CAD build for the part. Positions are in the model's coordinates, mm. Face numbers are marked on the shaded views. A direction names the side the tool comes from. Coordinates: 2 decimals unless noted, no trailing zeros. Order: outer loops, then holes, each group sorted by start corner. A loop starts at its lowest first (then second) coordinate and runs counter-clockwise, first axis right, second up. Notation, with made-up numbers: (43.25, -34.75) - (72.25, -34.75) arc R22 cw to (72.25, -3.75) - close; hole circle Ø7 at (-12.75, -10.5). An arc over 180 degrees is marked (long way). Return JSON: item names as keys, results as strings.
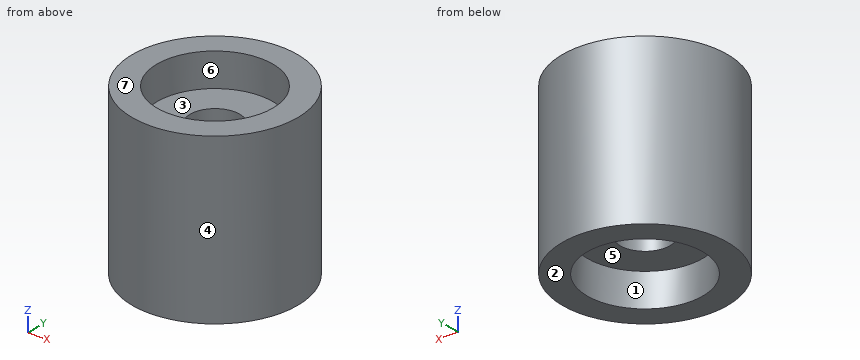
from build123d import *

# Parameters (mm, degrees)
SKETCH1_R           = 5
BOSS_EXTRUDE1_DEPTH = 10
SKETCH2_R           = 3.5
CUT_EXTRUDE1_DEPTH  = 2
SKETCH3_R           = 3.5
CUT_EXTRUDE2_DEPTH  = 2
SKETCH4_R           = 1.5
CUT_EXTRUDE3_DEPTH  = 12


with BuildPart() as part:
    # Sketch1 → Boss-Extrude1 (new body)
    with BuildSketch(Plane.XY):
        Circle(SKETCH1_R)
    extrude(amount=BOSS_EXTRUDE1_DEPTH)

    # Sketch2 → Cut-Extrude1 (cut)
    with BuildSketch(Plane.XY):
        Circle(SKETCH2_R)
    extrude(amount=CUT_EXTRUDE1_DEPTH, mode=Mode.SUBTRACT)

    # Sketch3 → Cut-Extrude2 (cut)
    with BuildSketch(Plane.XY.offset(10)):
        Circle(SKETCH3_R)
    extrude(amount=-CUT_EXTRUDE2_DEPTH, mode=Mode.SUBTRACT)

    # Sketch4 → Cut-Extrude3 (cut)
    with BuildSketch(Plane.XY.offset(10)):
        Circle(SKETCH4_R)
    extrude(amount=-CUT_EXTRUDE3_DEPTH, mode=Mode.SUBTRACT)


solid = part.part
Item 1: Band-saw the part on D-D, the plane y = -3.25. List the corners of the cut face in (x, z), then the cut area to 3 significant figures.
Findings below:
{"outline": "(-3.8, 0) - (-1.3, 0) - (-1.3, 2) - (1.3, 2) - (1.3, 0) - (3.8, 0) - (3.8, 10) - (1.3, 10) - (1.3, 8) - (-1.3, 8) - (-1.3, 10) - (-3.8, 10) - close", "area": "65.6 mm²"}
Item 2: Mould opens along Y. For the marked faces 4, 5, 6 and 7 say: released by +Y, released by -Y, zero draft, split by the parting line, or undercut.
Findings below:
{"face 4": "split by the parting line", "face 5": "undercut", "face 6": "undercut", "face 7": "zero draft"}
Item 3: Band-saw the part on A-A, the plane x = 0. List the corners of the cut face in (y, z).
Findings below:
{"outline": "(-5, 0) - (-3.5, 0) - (-3.5, 2) - (-1.5, 2) - (-1.5, 8) - (-3.5, 8) - (-3.5, 10) - (-5, 10) - close; (1.5, 2) - (3.5, 2) - (3.5, 0) - (5, 0) - (5, 10) - (3.5, 10) - (3.5, 8) - (1.5, 8) - close"}
Item 4: Band-saw the part on C-C, the plane z = 8.25. List the corners of the cut face in (x, y), then the cut area to 3 significant figures.
Findings below:
{"outline": "circle Ø10 at (0, 0); hole circle Ø7 at (0, 0)", "area": "40.1 mm²"}
Item 5: Drop flat-ended pins along their axis: P1, Ø2, axis at x = -1, y = -1.5, coming from the -Z side; P2, Ø2.5, axis at x = 0, y = 0, coming from the +Z side; P3, Ø1, axis at x = -3.5, z = 3.5, coming from the +Y side; P4, Ø1, axis at x = 2, z = 4.5, coming from the +Y side. Give the stop position or say it passes through.
Findings below:
{"P1": "stops at z = 2", "P2": "passes through", "P3": "stops at y = 4", "P4": "stops at y = 4.77"}
Item 6: Which spindle directions (+Z, -Z, +X, -X, +Y, -Y) get a long thin tool onto all of the face, cutting with end or side? Do the marked faces 1, 2 and 3. Say none if no direction does.
Findings below:
{"face 1": "-Z", "face 2": "-Z, +X, -X, +Y, -Y", "face 3": "+Z"}
Item 7: Wall check: L1, parallel to Y at x = 0, z = 0.95; L2, parallel to Y at x = 0, z = 4.5; L3, parallel to Z at x = 0.5, y = -2. Give the ranges that are in metal, low to high. Write a range as [from, to].
Findings below:
{"L1": "y = [-5, -3.5], [3.5, 5]", "L2": "y = [-5, -1.5], [1.5, 5]", "L3": "z = [2, 8]"}
